The figure shows three views and two pictorial views of one solid part (mm, origin at its lowest corner). Answer the questions. A direction names the side the tool comes from. Give positions to 0.01 mm unless a question says otherwise; leave off trailing zeros. Order: outer loops, then holes, each group sorted by start corner. A loop starts at its lowest first (then second) coordinate and runs counter-clockwise, first axis right, second up. Notation, with made-up numbers: (-21, -5) - (14, -5) arc R19 cw to (14, 1) - close; hole circle Ø3 at (69, 72). An arc over 180 degrees is marked (long way). Use a Markdown table: item, result. Add a question column.
1. A cutting plane is placed at B-B on y = 5. Determine the outline of the cut face in (x, z), and give its area (3 significant figures).
2. A cutting plane is placed at D-D on y = 1.25. Determine the outline of the cut face in (x, z).
3. A cutting plane is placed at C-C on z = 0.8. Determine the outline of the cut face in (x, y).
4. A cutting plane is placed at A-A on x = 8.5. Determine the outline of the cut face in (y, z).
5. For a pull along X with two mould halves and no side action, classify the marked faces 5, 6, 7 and 8 as released by +X, released by -X, zero draft, split by the parting line, or undercut.
6. Which of the six approach directions +Z, -Z, +X, -X, +Y, -Y give full straight-line access (tool end or side, diameter ignored) to the marked faces 1, 2, 3 and 4?
7. Consider L1, parallel to X at y = 5, z = 1.35; L2, parallel to Y at x = 8.5, z = 0.85; L3, parallel to X at y = 8, z = 0.75. Determine where each line is inside the solid, lowest interval first.
8. Flat-ended cylindrical pins translate along their axes: P1, Ø0.9, axis at x = 15.5, z = 1.5, coming from the -Y side; P2, Ø0.9, axis at y = 8, z = 1, coming from the -X side; P3, Ø1.5, axis at x = 15, z = 2.5, coming from the +Y side; P4, Ø2.5, axis at x = 8.5, y = 5, coming from the +Z side. Find the tip coordinate at first contact, or state that the pin passes through.
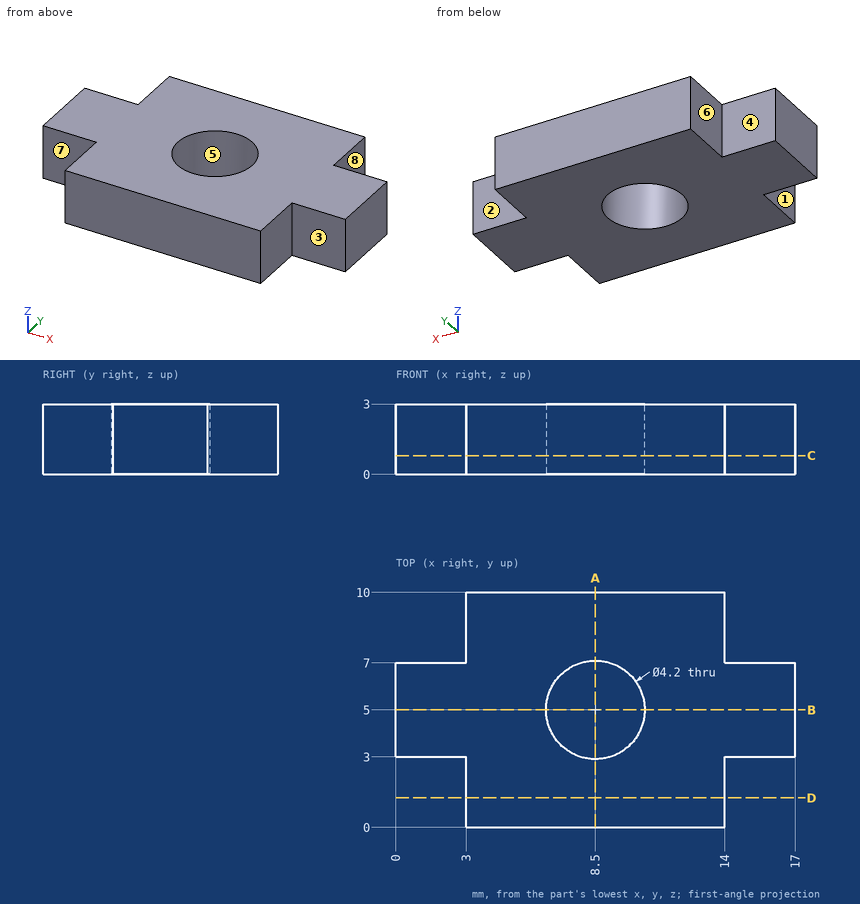
Output values:
| question | item | result |
|---|---|---|
| 1 | outline | (0, 0) - (6.4, 0) - (6.4, 3) - (0, 3) - close; (10.6, 0) - (17, 0) - (17, 3) - (10.6, 3) - close |
| 1 | area | 38.4 mm² |
| 2 | outline | (3, 0) - (14, 0) - (14, 3) - (3, 3) - close |
| 3 | outline | (0, 3) - (3, 3) - (3, 0) - (14, 0) - (14, 3) - (17, 3) - (17, 7) - (14, 7) - (14, 10) - (3, 10) - (3, 7) - (0, 7) - close; hole circle Ø4.2 at (8.5, 5) |
| 4 | outline | (0, 0) - (2.9, 0) - (2.9, 3) - (0, 3) - close; (7.1, 0) - (10, 0) - (10, 3) - (7.1, 3) - close |
| 5 | face 5 | undercut |
| 5 | face 6 | released by -X |
| 5 | face 7 | zero draft |
| 5 | face 8 | released by +X |
| 6 | face 1 | +Z, -Z, -X, -Y |
| 6 | face 2 | +Z, -Z, +X, +Y |
| 6 | face 3 | +Z, -Z, +X, -Y |
| 6 | face 4 | +Z, -Z, -X, +Y |
| 7 | L1 | 0 to 6.4, 10.6 to 17 |
| 7 | L2 | 0 to 2.9, 7.1 to 10 |
| 7 | L3 | 3 to 14 |
| 8 | P1 | y = 3 |
| 8 | P2 | x = 3 |
| 8 | P3 | y = 7 |
| 8 | P4 | through |
